Can you work these out from the model? Positions are in its coordinate system, mm. A direction names the side the tool comes from. Coordinates: 2 decimals unless noted, no trailing zeros. Loops run counter-clockwise (first coordinate to the right, second up) from the corner with the lowest first, then second, coordinate; pieces in that order, holes last. Notation, with made-up numbers: (-21, 10) -> (11, 10) arc R34 ccw to (11, 41) -> close; hole circle Ø7 at (19, 6.5). An arc over 180 degrees is marked (long way). Put each result on its own line as item: value. Start each with the question number.
Item 1: If we section it at A-A on y = 17.5: Please give me the cut outline in (x, z), plus the area to 3 significant figures.
Item 2: If we section it at C-C on x = 117: Please give me the cut outline in (y, z).
Item 3: Please list where these lines run through material, in increasing order: L1, parallel to X at y = 26, z = 0; L2, parallel to X at y = 11.75, z = -6.5; L3, parallel to X at y = 22.75, z = -122. Write a range as from..to.
Item 4: For faces 4 (the flat face through (98, 10, 95)), 5 (the flat face through (-52, 0, -3)), which set-ups out of +Z, -Z, +X, -X, +Y, -Y let a thin tool reach every point of the face, with its end or its side?
Item 5: We'd pull the mould along X, two halves only. Please class faces 1 (the flat face through (223, 30, -94)), 2 (the cylindrical face through (10.99, 14.79, -249.76)), 3 (the flat face through (-95, 10, -98)): pulls with the +X half, pulls with the -X half, needs draft (parallel to the pull), parting line crosses it, or undercut.
Item 6: Will these pins go through, and if not, where does the flat tip stop? P1, Ø12, axis at x = 150.5, y = 16.5, coming from the -Z side; P2, Ø8, axis at y = 11, z = 8.5, coming from the -X side; P3, Ø4, axis at y = 4, z = -198.5, coming from the -X side; P4, Ø8, axis at x = 0, z = 0, coming from the +Y side.
Item 7: If we section it at B-B on z = -21.5: Please give me the cut outline in (x, y).
```python
from build123d import *

# Parameters (mm, degrees)
CROQUIS1_R              = 250
SALIENTE_EXTRUIR1_DEPTH = 10
CROQUIS2_R              = 250
CROQUIS2_R_2            = 240
SALIENTE_EXTRUIR2_DEPTH = 20
CROQUIS3_R              = 15
SALIENTE_EXTRUIR3_DEPTH = 15
CROQUIS4_R              = 5
CORTAR_EXTRUIR1_DEPTH   = 355.436171969
CROQUIS5_W              = 235.044023843
CROQUIS5_H              = 10
CROQUIS5_W_2            = 10
CROQUIS5_H_2            = 235.044023843
SALIENTE_EXTRUIR4_DEPTH = 15


with BuildPart() as part:
    # Croquis1 → Saliente-Extruir1 (new body)
    with BuildSketch(Plane(origin=(0, 0, 0), x_dir=(1, 0, 0), z_dir=(0, 1, 0))):
        with Locations(Location((0, 0, 0), (0, 0, 270))):
            Circle(CROQUIS1_R)
    extrude(amount=SALIENTE_EXTRUIR1_DEPTH)

    # Croquis2 → Saliente-Extruir2 (add)
    with BuildSketch(Plane(origin=(0, 10, 0), x_dir=(1, 0, 0), z_dir=(0, 1, 0))):
        with Locations(Location((0, 0, 0), (0, 0, 270))):
            Circle(CROQUIS2_R)
        with Locations(Location((0, 0, 0), (0, 0, 270))):
            Circle(CROQUIS2_R_2, mode=Mode.SUBTRACT)
    extrude(amount=SALIENTE_EXTRUIR2_DEPTH)

    # Croquis3 → Saliente-Extruir3 (add)
    with BuildSketch(Plane(origin=(0, 10, 0), x_dir=(1, 0, 0), z_dir=(0, 1, 0))):
        with Locations(Location((0, 0, 0), (0, 0, 270))):
            Circle(CROQUIS3_R)
    extrude(amount=SALIENTE_EXTRUIR3_DEPTH)

    # Croquis4 → Cortar-Extruir1 (cut, through all)
    with BuildSketch(Plane(origin=(0, 25, 0), x_dir=(1, 0, 0), z_dir=(0, 1, 0))):
        with Locations(Location((0, 0, 0), (0, 0, 270))):
            Circle(CROQUIS4_R)
    extrude(amount=-CORTAR_EXTRUIR1_DEPTH, mode=Mode.SUBTRACT)

    # Croquis5 → Saliente-Extruir4 (add)
    with BuildSketch(Plane(origin=(0, 10, 0), x_dir=(1, 0, 0), z_dir=(0, 1, 0))):
        with Locations((126.662657579, 0)):
            Rectangle(CROQUIS5_W, CROQUIS5_H)
        with Locations((0, -126.662657579)):
            Rectangle(CROQUIS5_W_2, CROQUIS5_H_2)
        with Locations((-126.662657579, 0)):
            Rectangle(CROQUIS5_W, CROQUIS5_H)
        with Locations((0, 126.662657579)):
            Rectangle(CROQUIS5_W_2, CROQUIS5_H_2)
    extrude(amount=SALIENTE_EXTRUIR4_DEPTH)


solid = part.part
```
Solutions:
1. outline: circle Ø500 at (0, 0); hole (-239.95, -5) arc R240 ccw to (-5, -239.95) -> (-5, -14.14) arc R15 cw to (-14.14, -5) -> close; hole (-239.95, 5) -> (-14.14, 5) arc R15 cw to (-5, 14.14) -> (-5, 239.95) arc R240 ccw to start; hole circle Ø10 at (0, 0); hole (5, -239.95) arc R240 ccw to (239.95, -5) -> (14.14, -5) arc R15 cw to (5, -14.14) -> close; hole (5, 14.14) arc R15 cw to (14.14, 5) -> (239.95, 5) arc R240 ccw to (5, 239.95) -> close
1. area: 25,000 mm^2
2. outline: (0, -220.93) -> (30, -220.93) -> (30, -209.55) -> (10, -209.55) -> (10, -5) -> (25, -5) -> (25, 5) -> (10, 5) -> (10, 209.55) -> (30, 209.55) -> (30, 220.93) -> (0, 220.93) -> close
3. L1: -250..-240, 240..250
3. L2: -249.92..-239.91, -13.52..13.52, 239.91..249.92
3. L3: -218.21..-206.68, -5..5, 206.68..218.21
4. face 4: +Y
4. face 5: +Z, -Z, +X, -X, -Y
5. face 1: needs draft
5. face 2: parting line crosses it
5. face 3: undercut
6. P1: z = -204.01
6. P2: x = -249.96
6. P3: x = -154.56
6. P4: through
7. outline: (-249.07, 0) -> (249.07, 0) -> (249.07, 30) -> (239.04, 30) -> (239.04, 10) -> (5, 10) -> (5, 25) -> (-5, 25) -> (-5, 10) -> (-239.04, 10) -> (-239.04, 30) -> (-249.07, 30) -> close
